```python
from build123d import *

# Parameters (mm, degrees)
SKETCH1_W           = 120
SKETCH1_H           = 50
SKETCH1_R           = 1.6
BOSS_EXTRUDE1_DEPTH = 3
SKETCH2_R           = 1.55
SKETCH2_W           = 23.5
SKETCH2_H           = 12.5
CUT_EXTRUDE1_DEPTH  = 10
CUT_EXTRUDE2_DEPTH  = 10
FILLET1_R           = 4
FILLET2_R           = 0.5


with BuildPart() as part:
    # Sketch1 → Boss-Extrude1 (new body)
    with BuildSketch(Plane(origin=(0, 0, 0), x_dir=(1, 0, 0), z_dir=(0, 1, 0))):
        Rectangle(SKETCH1_W, SKETCH1_H)
        with Locations(Location((-54, 19, 0), (0, 0, 270))):
            Circle(SKETCH1_R, mode=Mode.SUBTRACT)
        with Locations(Location((54, 19, 0), (0, 0, 270))):
            Circle(SKETCH1_R, mode=Mode.SUBTRACT)
        with Locations(Location((54, -19, 0), (0, 0, 270))):
            Circle(SKETCH1_R, mode=Mode.SUBTRACT)
        with Locations(Location((-54, -19, 0), (0, 0, 270))):
            Circle(SKETCH1_R, mode=Mode.SUBTRACT)
    extrude(amount=BOSS_EXTRUDE1_DEPTH)

    # Sketch2 → Cut-Extrude1 (cut)
    with BuildSketch(Plane(origin=(0, 3, 0), x_dir=(1, 0, 0), z_dir=(0, 1, 0))):
        with Locations(Location((44, 17.5, 0), (0, 0, 270))):
            Circle(SKETCH2_R)
        with Locations(Location((44, -17.5, 0), (0, 0, 270))):
            Circle(SKETCH2_R)
        with BuildLine():
            Line((-54.73176855, 7.05), (-54.73176855, 8.55))
            ThreePointArc((-54.73176855, 8.55), (-53.15676855, 10.125), (-51.58176855, 8.55))
            Line((-51.58176855, 8.55), (-51.58176855, 7.05))
            ThreePointArc((-51.58176855, 7.05), (-53.15676855, 5.475), (-54.73176855, 7.05))
        make_face()
        with BuildLine():
            Line((-51.58176855, -7.05), (-51.58176855, -8.55))
            ThreePointArc((-51.58176855, -8.55), (-53.15676855, -10.125), (-54.73176855, -8.55))
            Line((-54.73176855, -8.55), (-54.73176855, -7.05))
            ThreePointArc((-54.73176855, -7.05), (-53.15676855, -5.475), (-51.58176855, -7.05))
        make_face()
        Rectangle(SKETCH2_W, SKETCH2_H)
        with BuildLine():
            Line((-5, 17.476998697), (5, 17.476998697))
            ThreePointArc((5, 17.476998697), (9, 13.476998697), (5, 9.476998697))
            Line((5, 9.476998697), (-5, 9.476998697))
            ThreePointArc((-5, 9.476998697), (-9, 13.476998697), (-5, 17.476998697))
        make_face()
        with BuildLine():
            Line((-14.5, 1.1), (-13.5, 1.1))
            ThreePointArc((-13.5, 1.1), (-12.4, 0), (-13.5, -1.1))
            Line((-13.5, -1.1), (-14.5, -1.1))
            ThreePointArc((-14.5, -1.1), (-15.6, 0), (-14.5, 1.1))
        make_face()
        with BuildLine():
            Line((13.5, 1.1), (14.5, 1.1))
            ThreePointArc((14.5, 1.1), (15.6, 0), (14.5, -1.1))
            Line((14.5, -1.1), (13.5, -1.1))
            ThreePointArc((13.5, -1.1), (12.4, 0), (13.5, 1.1))
        make_face()
    extrude(amount=-CUT_EXTRUDE1_DEPTH, mode=Mode.SUBTRACT)

    # Sketch4 → Cut-Extrude2 (cut)
    with BuildSketch(Plane(origin=(0, 3, 0), x_dir=(1, 0, 0), z_dir=(0, 1, 0))):
        with BuildLine():
            Line((-36.5, -25), (36.5, -25))
            ThreePointArc((36.5, -25), (0, -20.158240592), (-36.5, -25))
        make_face()
        with BuildLine():
            Line((-36.5, 25), (36.5, 25))
            ThreePointArc((36.5, 25), (0, 20.158240592), (-36.5, 25))
        make_face()
    extrude(amount=-CUT_EXTRUDE2_DEPTH, mode=Mode.SUBTRACT)

    # Fillet1
    fillet1_edges = [part.edges().sort_by_distance(p)[0] for p in [
        (60, 1.5, 25),
        (-60, 1.5, 25),
        (-60, 1.5, -25),
        (60, 1.5, -25),
    ]]
    fillet(fillet1_edges, radius=FILLET1_R)

    # Fillet2
    fillet2_edges = [part.edges().sort_by_distance(p)[0] for p in [
        (46.25, 0, 25),
        (46.25, 3, 25),
        (-46.25, 0, -25),
        (-46.25, 3, -25),
        (-36.5, 1.5, -25),
        (36.5, 1.5, -25),
        (0, 0, 20.158240592),
        (0, 3, 20.158240592),
        (0, 0, -20.158240592),
        (0, 3, -20.158240592),
        (-46.25, 0, 25),
        (-46.25, 3, 25),
        (-60, 0, 0),
        (46.25, 0, -25),
        (60, 0, 0),
        (58.828427125, 0, -23.828427125),
        (-58.828427125, 0, -23.828427125),
        (58.828427125, 0, 23.828427125),
        (-58.828427125, 0, 23.828427125),
        (-60, 3, 0),
        (60, 3, 0),
        (46.25, 3, -25),
        (58.828427125, 3, -23.828427125),
        (-58.828427125, 3, -23.828427125),
        (58.828427125, 3, 23.828427125),
        (-58.828427125, 3, 23.828427125),
    ]]
    fillet(fillet2_edges, radius=FILLET2_R)


solid = part.part
```
Read the model definition and answer for the solid it produces. Units are mm, in the model's axes. A direction names the side the tool comes from. Give positions to 0.01 mm unless a question says otherwise; leave off trailing zeros. Order: outer loops, then holes, each group sorted by start corner. A loop starts at its lowest first (then second) coordinate and runs counter-clockwise, first axis right, second up. Notation, with made-up numbers: (-24, 61) -> (15, 61) arc R31 ccw to (15, 100) -> close; hole circle Ø6 at (49, 24). An arc over 180 degrees is marked (long way). One line per item, written item: value. Start each with the question number.
(1) The part is cut by section C-C (y = 1.55). State how many separate pieces and enclosed holes the cut face has, and give its area (3 significant figures).
(2) The part is cut by section A-A (z = -3). Determine the outline of the cut face in (x, y).
(3) For a pull along X with two mould halves and no side action, classify faces 3 (the flat face through (-46, 1, 25)), 4 (the cylindrical face through (-53.122, 1.521, -5.475)), 5 (the cylindrical face through (-58.859, 1.514, -23.797)), 6 (the cylindrical face through (-15.6, 1.5, 0)) as released by +X, released by -X, zero draft, split by the parting line, or undercut.
(4) A tool of negligible diameter and unlimited length cuts with its end or side. For faces 1 (the flat face through (-46, 1, -25)), 2 (the flat face through (0, 2, -6.25)), from which of +Z, -Z, +X, -X, +Y, -Y can it reach the whole face along a straight path? Write none if from no direction.
(5) Straight lines are drawn through the part: L1, parallel to Z at x = -6, y = 2.5; L2, parallel to Z at x = 53.5, y = 1.9; L3, parallel to X at y = 2.2, z = -1. For each, find the intervals that lie inside material, in ascending order.
(6) The part is cut by section B-B (x = 44). Determine the outline of the cut face in (y, z).
(7) Flat-ended cylindrical pins translate along their axes: P1, Ø1.9, axis at x = 44, z = -17.5, coming from the +Y side; P2, Ø0.9, axis at x = 0.5, y = 1, coming from the +Z side; P3, Ø0.5, axis at x = 14, y = 2, coming from the +Z side; P4, Ø3.5, axis at x = 54, z = -19, coming from the -Y side. Find the tip coordinate at first contact, or state that the pin passes through.
Taken from the geometry:
1. separate pieces: 1
1. enclosed holes: 12
1. area: 5,010 mm^2
2. outline: (-60, 0.5) arc R0.5 ccw to (-59.5, 0) -> (-11.75, 0) -> (-11.75, 3) -> (-59.5, 3) arc R0.5 ccw to (-60, 2.5) -> close; (11.75, 0) -> (59.5, 0) arc R0.5 ccw to (60, 0.5) -> (60, 2.5) arc R0.5 ccw to (59.5, 3) -> (11.75, 3) -> close
3. face 3: zero draft
3. face 4: undercut
3. face 5: released by -X
3. face 6: undercut
4. face 1: -Z, +X, -X, +Y, -Y
4. face 2: +Y, -Y
5. L1: -20.29 to -17.35, -9.6 to -6.25, 6.25 to 20.29
5. L2: -25 to -20.52, -17.48 to 17.48, 20.52 to 25
5. L3: -60 to -14.96, -13.04 to -11.75, 11.75 to 13.04, 14.96 to 60
6. outline: (0, -24.5) arc R0.5 ccw to (0.5, -25) -> (2.5, -25) arc R0.5 ccw to (3, -24.5) -> (3, -19.05) -> (0, -19.05) -> close; (0, -15.95) -> (3, -15.95) -> (3, 15.95) -> (0, 15.95) -> close; (0, 19.05) -> (3, 19.05) -> (3, 24.5) arc R0.5 ccw to (2.5, 25) -> (0.5, 25) arc R0.5 ccw to (0, 24.5) -> close
7. P1: through
7. P2: z = 20.16
7. P3: z = 20.89
7. P4: y = 0
